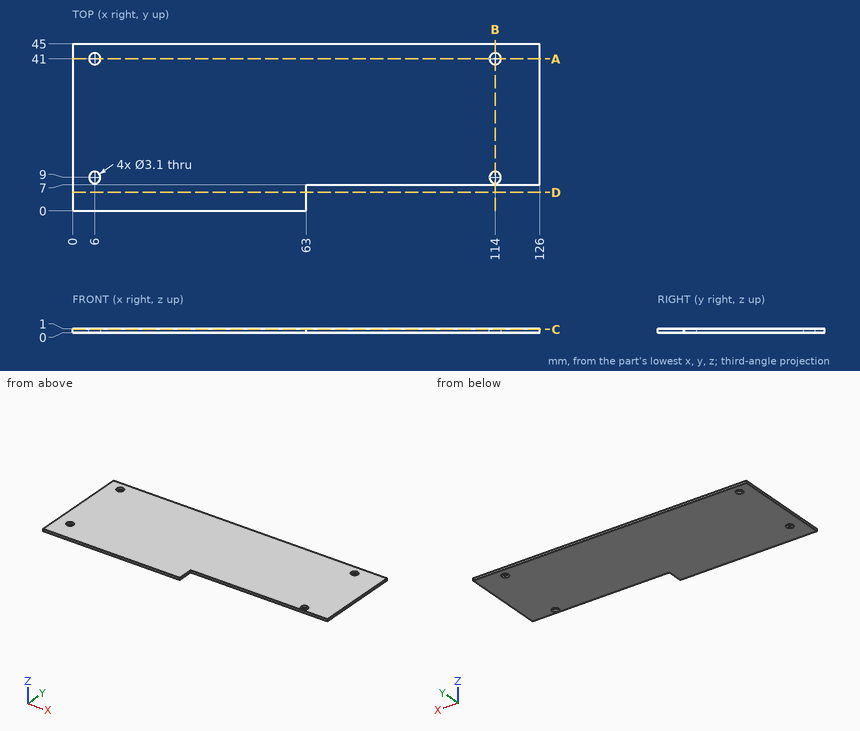
For this review, use the dimensioned drawing (mm, ordinates from the lowest corner) and the shaded views. Coordinates: 2 decimals unless noted, no trailing zeros. Loops run counter-clockwise (first coordinate to the right, second up) from the corner with the lowest first, then second, coordinate; pieces in that order, holes last.
1. Add section C-C, the plane z = 0.85. Give the boundary of the cut face in (x, y).
2. For line 1 (X direction, y = 41, z = 0.5); line 2 (Y direction, x = 6, z = 0.25); line 3 (Y direction, x = 114, z = 0.3), list the stretches that pass through material, from the lowest coordinate up.
3. Add section A-A, the plane y = 41. Give the boundary of the cut face in (x, z), then the cut area to 3 significant figures.
4. Add section B-B, the plane x = 114. Give the boundary of the cut face in (y, z), then the cut area to 3 significant figures.
5. Add section D-D, the plane y = 5. Give the boundary of the cut face in (x, z), then the cut area to 3 significant figures.
Result:
1. outline: (0, 0) - (63, 0) - (63, 7) - (126, 7) - (126, 45) - (0, 45) - close; hole circle Ø3.1 at (6, 9); hole circle Ø3.1 at (6, 41); hole circle Ø3.1 at (114, 9); hole circle Ø3.1 at (114, 41)
2. line 1: x = 0 to 4.45, 7.55 to 112.45, 115.55 to 126
2. line 2: y = 0 to 7.45, 10.55 to 39.45, 42.55 to 45
2. line 3: y = 7 to 7.45, 10.55 to 39.45, 42.55 to 45
3. outline: (0, 0) - (4.45, 0) - (4.45, 1) - (0, 1) - close; (7.55, 0) - (112.45, 0) - (112.45, 1) - (7.55, 1) - close; (115.55, 0) - (126, 0) - (126, 1) - (115.55, 1) - close
3. area: 120 mm2
4. outline: (7, 0) - (7.45, 0) - (7.45, 1) - (7, 1) - close; (10.55, 0) - (39.45, 0) - (39.45, 1) - (10.55, 1) - close; (42.55, 0) - (45, 0) - (45, 1) - (42.55, 1) - close
4. area: 31.8 mm2
5. outline: (0, 0) - (63, 0) - (63, 1) - (0, 1) - close
5. area: 63.0 mm2
